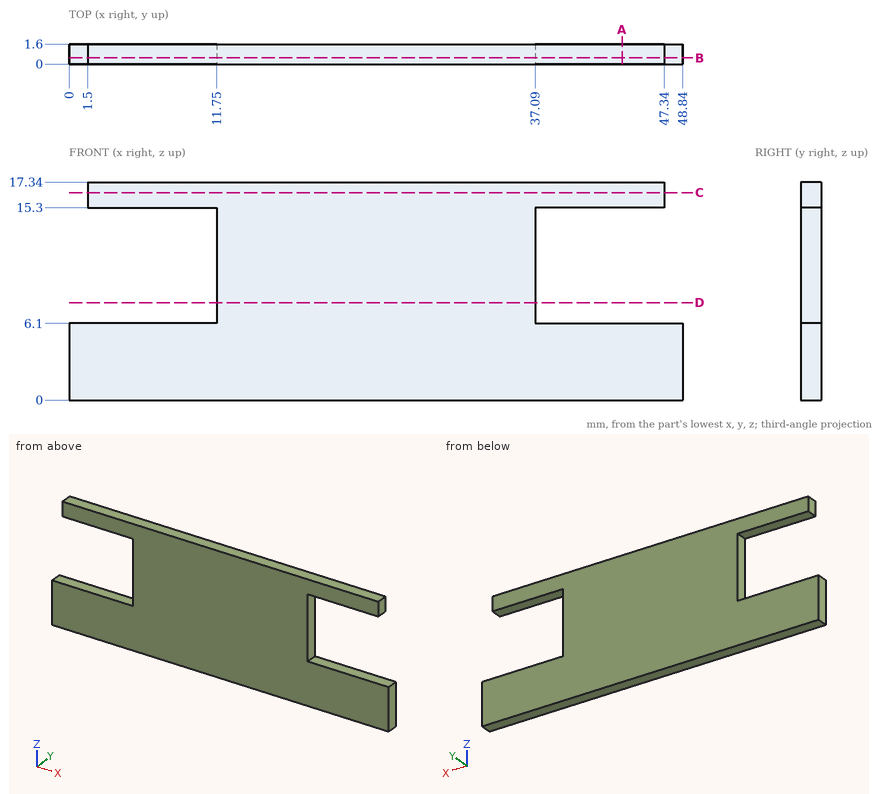
Part print with two shaded views. Sizes in mm from the minimum x, y, z corner. Coordinates: 2 decimals unless noted, no trailing zeros. Order: outer loops, then holes, each group sorted by start corner. A loop starts at its lowest first (then second) coordinate and runs counter-clockwise, first axis right, second up. Notation, with made-up numbers: (78.25, 7) - (90.25, 7) arc R32 cw to (90.25, 44) - close; hole circle Ø1 at (-25, 73). An arc over 180 degrees is marked (long way). Write item = value, one per line. Start each with the question number.
1) Saw through at B-B on y = 0.5. Write the cut outline in (x, z), then the cut area to 3 significant figures.
2) Flat gauge pins, fed straight in: pin 1 Ø8 at (x, z) = (43, 11.5) entering from +Y; pin 2 Ø0.5 at (y, z) = (0.5, 9.5) entering from -X; pin 3 Ø0.8 at (y, z) = (0.5, 12) entering from +X. Where does each tip first touch, or does it go through?
3) Saw through at C-C on z = 16.5. Write the cut outline in (x, y), then the cut area to 3 significant figures.
4) Saw through at A-A on x = 44. Write the cut outline in (y, z), then the cut area to 3 significant figures.
5) Saw through at D-D on z = 7.75. Write the cut outline in (x, y).
6) Wall check: line 1 along Z through (x, y) = (7.5, 0.6); line 2 along X through (y, z) = (0.45, 12); line 3 along X through (y, z) = (0.25, 16.5). Give the ranges that are in metal, low to high. Write a range as from..to.
From the geometry:
q1.outline = (0, 0) - (48.84, 0) - (48.84, 6.1) - (37.09, 6.1) - (37.09, 15.3) - (47.34, 15.3) - (47.34, 17.34) - (1.5, 17.34) - (1.5, 15.3) - (11.75, 15.3) - (11.75, 6.1) - (0, 6.1) - close
q1.area = 625 mm^2
q2.pin_1 = 1.6
q2.pin_2 = 11.75
q2.pin_3 = 37.09
q3.outline = (1.5, 0) - (47.34, 0) - (47.34, 1.6) - (1.5, 1.6) - close
q3.area = 73.3 mm^2
q4.outline = (0, 0) - (1.6, 0) - (1.6, 6.1) - (0, 6.1) - close; (0, 15.3) - (1.6, 15.3) - (1.6, 17.34) - (0, 17.34) - close
q4.area = 13.0 mm^2
q5.outline = (11.75, 0) - (37.09, 0) - (37.09, 1.6) - (11.75, 1.6) - close
q6.line_1 = 0..6.1, 15.3..17.34
q6.line_2 = 11.75..37.09
q6.line_3 = 1.5..47.34
